```python
from build123d import *

# Parameters (mm, degrees)
F0_R          = 500
F3_DEPTH      = 1000
F5_DEPTH      = 500.001
F5_DEPTH_BACK = 500.001


with BuildPart() as f3:
    # F0 (on Top) → F3 (new body, through all)
    with BuildSketch(Plane.XY):
        Circle(F0_R)
    extrude(amount=F3_DEPTH)


with BuildPart() as f5:
    # F4 (on Front) → F5 (new body, two sides)
    with BuildSketch(Plane.XZ) as f5_sk:
        Polygon((0, 1000), (500, 0), (500, 1000), align=None)
    extrude(amount=-F5_DEPTH)
    extrude(f5_sk.sketch, amount=F5_DEPTH_BACK)


with BuildPart() as f6_1:
    # F6: instance of F5
    add(f5.part.mirror(Plane.YZ))


with BuildPart() as f3_1:
    add(f3.part)

    # F7: cut F5, F6_1
    add(f5.part, mode=Mode.SUBTRACT)
    add(f6_1.part, mode=Mode.SUBTRACT)


solid = f3_1.part
```
Verification items for the finished model (mm, model axes). Round coordinates to 2 decimals unless told otherwise and drop trailing zeros. Order: outer loops, then holes, each group sorted by start corner. A loop starts at its lowest first (then second) coordinate and runs counter-clockwise, first axis right, second up. Notation, with made-up numbers: (12, 67.25) - (41, 67.25) arc R18 cw to (41, 76.25) - close; hole circle Ø5 at (-8, 1). An arc over 180 degrees is marked (long way). Use CSV: the item, a comma, the result in double quotes.
(1) Section check D-D on y = -184.5. Record the boundary of the cut face in (x, z).
Entries:
outline,"(-464.71, 0) - (464.71, 0) - (464.71, 70.57) - (0, 1000) - (-464.71, 70.57) - close"
(2) Section check A-A on y = 42.5. Record the boundary of the cut face in (x, z), and give its area (3 significant figures).
Entries:
outline,"(-498.19, 0) - (498.19, 0) - (498.19, 3.62) - (0, 1000) - (-498.19, 3.62) - close"
area,"500,000 mm^2"
(3) Thickness scan on probe 1 along X at (y, z) = (-160.5, 746.5); probe 2 along X at (y, z) = (300.5, 287.5); probe 3 along Y at (x, z) = (-112, 748.5). Record the ranges inside material, lowest first. Write a range as from..to.
Entries:
probe 1,"-126.75..126.75"
probe 2,"-356.25..356.25"
probe 3,"-487.29..487.29"
(4) Section check C-C on x = 83. Record the boundary of the cut face in (y, z), and give its area (3 significant figures).
Entries:
outline,"(-493.06, 0) - (493.06, 0) - (493.06, 834) - (-493.06, 834) - close"
area,"822,000 mm^2"
(5) Gauge pin test, flat ends, axial feed: pin 1 Ø8 at (y, z) = (-40, 716) entering from +X; pin 2 Ø10 at (x, y) = (172.5, 377.5) entering from +Z; pin 3 Ø12 at (x, y) = (313.5, 156.5) entering from +Z. Record the tip position at first contact, or that the pin passes through.
Entries:
pin 1,"x = 144"
pin 2,"z = 665"
pin 3,"z = 385"
(6) Section check B-B on z = 585. Record the boundary of the cut face in (x, y), and give its area (3 significant figures).
Entries:
outline,"(-207.5, -454.91) arc R500 ccw to (207.5, -454.91) - (207.5, 454.91) arc R500 ccw to (-207.5, 454.91) - close"
area,"403,000 mm^2"
